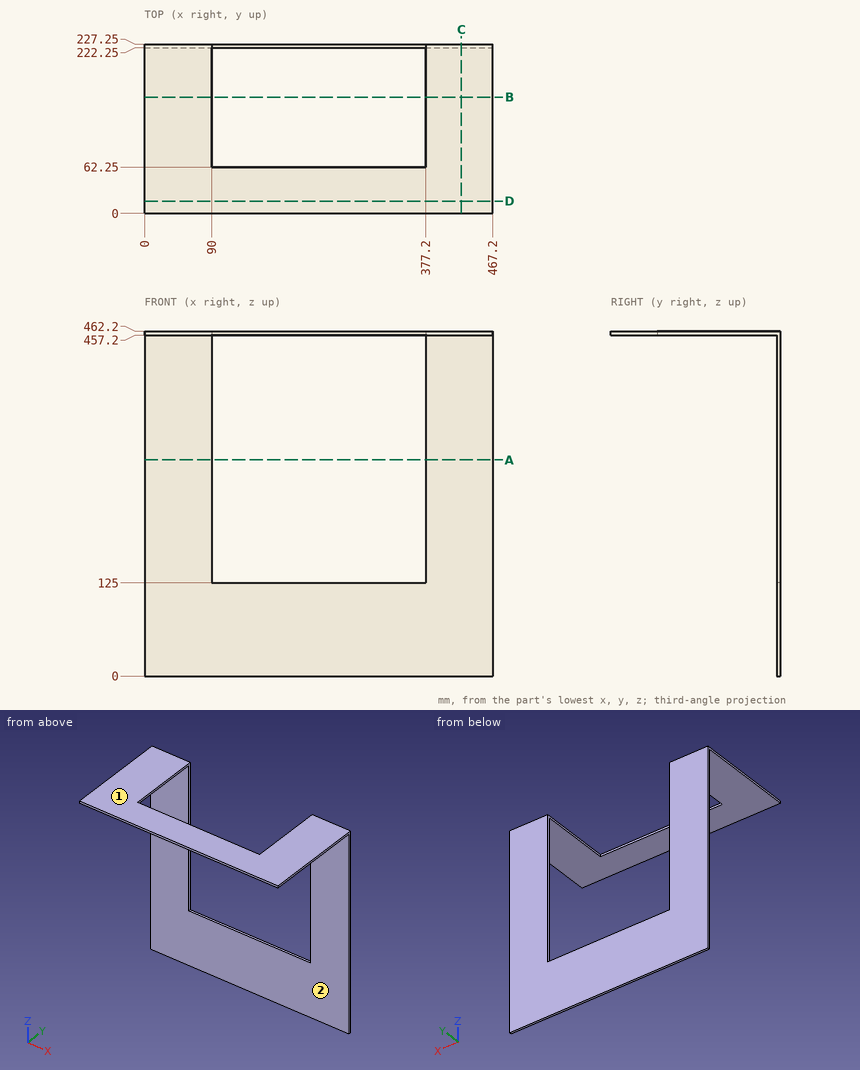
Study the drawing (mm; zero at the part's minimum x, y, z) and answer. A direction names the side the tool comes from. Give positions to 0.01 mm unless a question says otherwise; leave off trailing zeros. Write each loop counter-clockwise with the first axis right and the second up, starting at its lowest first coordinate (ties: lowest second). Pieces come first, ordered by that corner, then holes. Notation, with made-up numbers: (18.5, -31) -> (67.5, -31) arc R10 ccw to (67.5, -14) -> close; hole circle Ø11 at (42, 16). An arc over 180 degrees is marked (long way). Answer as a JSON object with one key per item and string values. Group by question number.
1) Find section C-C (x = 425). Write down the section's boundary in (y, z), and give its area (3 significant figures).
2) Each of these flat-tipped pins is pushed along its axis until it touches: P1, Ø2.5, axis at x = 252, z = 459.5, coming from the +Y side; P2, Ø2.5, axis at x = 239, y = 225, coming from the +Z side. Where does it stop, or does it pass through?
3) A tool of negligible diameter and unlimited length cuts with its end or side. For the marked faces 1 and 2, from which of +Z, -Z, +X, -X, +Y, -Y can it reach the whole face along a straight path? Write none if from no direction.
4) Find section D-D (y = 16.5). Write down the section's boundary in (x, z), and give its area (3 significant figures).
5) Consider L1, parallel to Y at x = 445.5, z = 175; L2, parallel to Z at x = 392.5, y = 149. Determine where each line is inside the solid, lowest interval first. Write a range as from..to.
6) Find section B-B (y = 156). Write down the section's boundary in (x, z), and give its area (3 significant figures).
7) Find section A-A (z = 290). Write down the section's boundary in (x, y).
Values follow:
{
 "1": {"outline": "(0, 457.2) -> (222.25, 457.2) -> (222.25, 0) -> (227.25, 0) -> (227.25, 462.2) -> (0, 462.2) -> close", "area": "3,420 mm2"},
 "2": {"P1": "stops at y = 62.25", "P2": "stops at z = 125"},
 "3": {"face 1": "+Z, +X, -X, +Y, -Y", "face 2": "-Z, +X, -X, -Y"},
 "4": {"outline": "(0, 457.2) -> (467.2, 457.2) -> (467.2, 462.2) -> (0, 462.2) -> close", "area": "2,340 mm2"},
 "5": {"L1": "y = 222.25..227.25", "L2": "z = 457.2..462.2"},
 "6": {"outline": "(0, 457.2) -> (90, 457.2) -> (90, 462.2) -> (0, 462.2) -> close; (377.2, 457.2) -> (467.2, 457.2) -> (467.2, 462.2) -> (377.2, 462.2) -> close", "area": "900 mm2"},
 "7": {"outline": "(0, 222.25) -> (90, 222.25) -> (90, 227.25) -> (0, 227.25) -> close; (377.2, 222.25) -> (467.2, 222.25) -> (467.2, 227.25) -> (377.2, 227.25) -> close"}
}
